from build123d import *

# Parameters (mm, degrees)
BOSS_EXTRUDE1_DEPTH = 15
FILLET1_R           = 5
FILLET2_R           = 1.5
SKETCH2_W           = 25
SKETCH2_H           = 5
CUT_EXTRUDE1_DEPTH  = 16
SKETCH3_R           = 1.6
CUT_EXTRUDE2_DEPTH  = 28.292857857
SKETCH4_R           = 3
CUT_EXTRUDE3_DEPTH  = 17.292858


with BuildPart() as part:
    # Sketch1 → Boss-Extrude1 (new body)
    with BuildSketch(Plane(origin=(0, 0, 0), x_dir=(1, 0, 0), z_dir=(0, 1, 0))):
        with BuildLine():
            ThreePointArc((-76.314992177, 5), (-35, 22.292857857), (6.314992177, 5))
            Line((6.314992177, 5), (14.314992177, 5))
            Line((14.314992177, 5), (14.314992177, 0))
            Line((14.314992177, 0), (0, 0))
            ThreePointArc((0, 0), (-35, 14.292857857), (-70, 0))
            Line((-70, 0), (-84.314992177, 0))
            Line((-84.314992177, 0), (-84.314992177, 5))
            Line((-84.314992177, 5), (-76.314992177, 5))
        make_face()
        with BuildLine():
            Line((-50, 32.292857857), (-50, 20.319637169))
            ThreePointArc((-50, 20.319637169), (-35, 22.292857857), (-20, 20.319637169))
            Line((-20, 20.319637169), (-20, 32.292857857))
            Line((-20, 32.292857857), (-50, 32.292857857))
        make_face()
    extrude(amount=BOSS_EXTRUDE1_DEPTH)

    # Fillet1
    fillet1_edges = [part.edges().sort_by_distance(p)[0] for p in [
        (-50, 7.5, -20.319637169),
        (-20, 7.5, -20.319637169),
        (6.314992177, 7.5, -5),
        (-76.314992177, 7.5, -5),
    ]]
    fillet(fillet1_edges, radius=FILLET1_R)

    # Fillet2
    fillet2_edges = [part.edges().sort_by_distance(p)[0] for p in [
        (14.314992177, 7.5, -5),
        (14.314992177, 7.5, 0),
        (-84.314992177, 7.5, 0),
        (-84.314992177, 7.5, -5),
    ]]
    fillet(fillet2_edges, radius=FILLET2_R)

    # Sketch2 → Cut-Extrude1 (cut, through all)
    with BuildSketch(Plane(origin=(0, 15, 0), x_dir=(1, 0, 0), z_dir=(0, 1, 0))):
        with Locations((-35, 29.792857857)):
            Rectangle(SKETCH2_W, SKETCH2_H)
    extrude(amount=-CUT_EXTRUDE1_DEPTH, mode=Mode.SUBTRACT)

    # Sketch3 → Cut-Extrude2 (cut, through all)
    with BuildSketch(Plane(origin=(0, 0, -27.292857857), x_dir=(-1, 0, 0), z_dir=(0, 0, -1))):
        with Locations((35, 7.5)):
            Circle(SKETCH3_R)
    extrude(amount=-CUT_EXTRUDE2_DEPTH, mode=Mode.SUBTRACT)

    # Sketch4 → Cut-Extrude3 (cut)
    with BuildSketch(Plane.XY):
        with Locations((-35, 7.5)):
            Circle(SKETCH4_R)
    extrude(amount=-CUT_EXTRUDE3_DEPTH, mode=Mode.SUBTRACT)


solid = part.part
The model under review builds one solid part; all positions refer to its coordinate system, in mm. A direction names the side the tool comes from. Round coordinates to 2 decimals unless told otherwise and drop trailing zeros. Loops run counter-clockwise (first coordinate to the right, second up) from the corner with the lowest first, then second, coordinate; pieces in that order, holes last. Notation, with made-up numbers: M 26.25,-9.5 L 33.25,-9.5 A11 cw 33.25,5.5 Z; hole C 3,-29.75 d2. An arc over 180 degrees is marked long. Answer as a JSON object with one key per item and string values.
Item 1: Tool access review of faces 1 (the face through (-34, 6, -17.293)), 2 (the face through (-50, 7, -28)), 3 (the face through (-22.5, 8, -30)), 4 (the face through (11, 7, -5)): name each direction out of +Z, -Z, +X, -X, +Y, -Y from which nothing blocks a thin tool from reaching the whole face with its end or side.
Check sheet entries:
{"face 1": "+Z", "face 2": "-Z, -X, +Y, -Y", "face 3": "-Z, +Y, -Y", "face 4": "-Z, +X, +Y, -Y"}
Item 2: We need section B-B, the plane x = -35. State the section outline as (y, z) points.
Check sheet entries:
{"outline": "M 0,-27.29 L 5.9,-27.29 L 5.9,-17.29 L 4.5,-17.29 L 4.5,-14.29 L 0,-14.29 Z; M 9.1,-27.29 L 15,-27.29 L 15,-14.29 L 10.5,-14.29 L 10.5,-17.29 L 9.1,-17.29 Z"}
Item 3: We need section D-D, the plane z = -11. State the section outline as (x, y) points.
Check sheet entries:
{"outline": "M -69.39,0 L -52.84,0 L -52.84,15 L -69.39,15 Z; M -17.16,0 L -0.61,0 L -0.61,15 L -17.16,15 Z"}
Item 4: We need section C-C, the plane y = 1.75. State the section outline as (x, z) points (3 decimals).
Check sheet entries:
{"outline": "M -84.315,-3.5 A1.5 ccw -82.815,-5 L -78.357,-5 A5 cw -74.916,-6.372 A58 ccw -53.413,-19.293 A5 cw -50,-24.034 L -50,-32.293 L -47.5,-32.293 L -47.5,-27.293 L -22.5,-27.293 L -22.5,-32.293 L -20,-32.293 L -20,-24.034 A5 cw -16.587,-19.293 A58 ccw 4.916,-6.372 A5 cw 8.357,-5 L 12.815,-5 A1.5 ccw 14.315,-3.5 L 14.315,-1.5 A1.5 ccw 12.815,0 L 0,0 A50 cw -70,0 L -82.815,0 A1.5 ccw -84.315,-1.5 Z"}
Item 5: Clearance check with flat-ended pins moving along their axes: P1, Ø1.8, axis at x = -34, y = 8.5, coming from the +Z side; P2, Ø4, axis at y = 9.5, z = -30, coming from the +X side; P3, Ø1, axis at y = 7.5, z = -15, coming from the -X side. State where each tip first meets the part, or that it passes through.
Check sheet entries:
{"P1": "z = -17.29", "P2": "x = -20", "P3": "x = -64.04"}
Item 6: For line 1 along Y through (x, z) = (-35, -23); line 2 along Y through (x, z) = (-35, -15.8); line 3 along X through (y, z) = (0.75, -29.5), list the stretches that pass through material, from the lowest coordinate up.
Check sheet entries:
{"line 1": "0 to 5.9, 9.1 to 15", "line 2": "0 to 4.5, 10.5 to 15", "line 3": "-50 to -47.5, -22.5 to -20"}
